The listing builds one solid part. Answer for the finished solid, in the listing's coordinates (mm). A direction names the side the tool comes from. Coordinates: 2 decimals unless noted, no trailing zeros. One line per item, written item: value. Start each with the question number.
```python
from build123d import *

# Parameters (mm, degrees)
SKETCH1_W           = 11.9
SKETCH1_H           = 5.95
BOSS_EXTRUDE1_DEPTH = 340
CUT_EXTRUDE1_DEPTH  = 341


with BuildPart() as part:
    # Sketch1 → Boss-Extrude1 (new body)
    with BuildSketch(Plane.XY):
        with BuildLine():
            Line((-4.350229073, 14.992640687), (-13.192640687, 14.992640687))
            ThreePointArc((-13.192640687, 14.992640687), (-14.465432893, 14.465432893), (-14.992640687, 13.192640687))
            Line((-14.992640687, 13.192640687), (-14.992640687, 4.350229073))
            Line((-14.992640687, 4.350229073), (-13.792640687, 4.350229073))
            ThreePointArc((-13.792640687, 4.350229073), (-13.085533906, 4.643122292), (-12.792640687, 5.350229073))
            Line((-12.792640687, 5.350229073), (-12.792640687, 8.460229073))
            Line((-12.792640687, 8.460229073), (-8.460229073, 8.460229073))
            Line((-8.460229073, 8.460229073), (-8.460229073, 12.792640687))
            Line((-8.460229073, 12.792640687), (-5.350229073, 12.792640687))
            ThreePointArc((-5.350229073, 12.792640687), (-4.643122292, 13.085533906), (-4.350229073, 13.792640687))
            Line((-4.350229073, 13.792640687), (-4.350229073, 14.992640687))
        make_face()
        with BuildLine():
            Line((-10.660229073, 13.792640687), (-12.792640687, 13.792640687))
            ThreePointArc((-12.792640687, 13.792640687), (-13.499747468, 13.499747468), (-13.792640687, 12.792640687))
            Line((-13.792640687, 12.792640687), (-13.792640687, 10.660229073))
            ThreePointArc((-13.792640687, 10.660229073), (-13.499747468, 9.953122292), (-12.792640687, 9.660229073))
            Line((-12.792640687, 9.660229073), (-10.660229073, 9.660229073))
            ThreePointArc((-10.660229073, 9.660229073), (-9.953122292, 9.953122292), (-9.660229073, 10.660229073))
            Line((-9.660229073, 10.660229073), (-9.660229073, 12.792640687))
            ThreePointArc((-9.660229073, 12.792640687), (-9.953122292, 13.499747468), (-10.660229073, 13.792640687))
        make_face(mode=Mode.SUBTRACT)
        Polygon((-5.95, 4.217588386), (-5.95, 5.95), (-4.217588386, 5.95), (-8.460229073, 10.192640687), (-8.460229073, 8.460229073), (-10.192640687, 8.460229073), align=None)
        with Locations((0, 2.975)):
            Rectangle(SKETCH1_W, SKETCH1_H)
        Polygon((8.460229073, 10.192640687), (4.217588386, 5.95), (5.95, 5.95), (5.95, 4.217588386), (10.192640687, 8.460229073), (8.460229073, 8.460229073), align=None)
        with BuildLine():
            Line((12.792640687, 8.460229073), (12.792640687, 5.350229073))
            ThreePointArc((12.792640687, 5.350229073), (13.085533906, 4.643122292), (13.792640687, 4.350229073))
            Line((13.792640687, 4.350229073), (14.992640687, 4.350229073))
            Line((14.992640687, 4.350229073), (14.992640687, 13.192640687))
            ThreePointArc((14.992640687, 13.192640687), (14.465432893, 14.465432893), (13.192640687, 14.992640687))
            Line((13.192640687, 14.992640687), (4.350229073, 14.992640687))
            Line((4.350229073, 14.992640687), (4.350229073, 13.792640687))
            ThreePointArc((4.350229073, 13.792640687), (4.643122292, 13.085533906), (5.350229073, 12.792640687))
            Line((5.350229073, 12.792640687), (8.460229073, 12.792640687))
            Line((8.460229073, 12.792640687), (8.460229073, 8.460229073))
            Line((8.460229073, 8.460229073), (12.792640687, 8.460229073))
        make_face()
        with BuildLine():
            ThreePointArc((9.660229073, 10.660229073), (9.953122292, 9.953122292), (10.660229073, 9.660229073))
            Line((10.660229073, 9.660229073), (12.792640687, 9.660229073))
            ThreePointArc((12.792640687, 9.660229073), (13.499747468, 9.953122292), (13.792640687, 10.660229073))
            Line((13.792640687, 10.660229073), (13.792640687, 12.792640687))
            ThreePointArc((13.792640687, 12.792640687), (13.499747468, 13.499747468), (12.792640687, 13.792640687))
            Line((12.792640687, 13.792640687), (10.660229073, 13.792640687))
            ThreePointArc((10.660229073, 13.792640687), (9.953122292, 13.499747468), (9.660229073, 12.792640687))
            Line((9.660229073, 12.792640687), (9.660229073, 10.660229073))
        make_face(mode=Mode.SUBTRACT)
    extrude(amount=-BOSS_EXTRUDE1_DEPTH)

    # Mirror1: part across plane


with BuildPart() as part_1:
    add(part.part)
    add(part.part.mirror(Plane(origin=(0, 0, -340), x_dir=(0, 0, 1), z_dir=(0, -1, 0))))

    # Sketch2 → Cut-Extrude1 (cut, through all)
    with BuildSketch(Plane.XY):
        with BuildLine():
            Line((-4.631549417, 3.075914498), (-3.16821753, 1.612582612))
            ThreePointArc((-3.16821753, 1.612582612), (-2.513764607, 2.513764607), (-1.612582612, 3.16821753))
            Line((-1.612582612, 3.16821753), (-3.075914498, 4.631549417))
            Line((-3.075914498, 4.631549417), (-4.631549417, 3.075914498))
        make_face()
        with BuildLine():
            Line((-3.16821753, 1.612582612), (-1.555634919, 0))
            Line((-1.555634919, 0), (0, 1.555634919))
            Line((0, 1.555634919), (-1.612582612, 3.16821753))
            ThreePointArc((-1.612582612, 3.16821753), (-2.513764607, 2.513764607), (-3.16821753, 1.612582612))
        make_face()
        with BuildLine():
            ThreePointArc((-3.16821753, 1.612582612), (-3.555, 0), (-3.16821753, -1.612582612))
            Line((-3.16821753, -1.612582612), (-1.555634919, 0))
            Line((-1.555634919, 0), (-3.16821753, 1.612582612))
        make_face()
        with BuildLine():
            Line((-4.631549417, -3.075914498), (-3.075914498, -4.631549417))
            Line((-3.075914498, -4.631549417), (-1.612582612, -3.16821753))
            ThreePointArc((-1.612582612, -3.16821753), (-2.513764607, -2.513764607), (-3.16821753, -1.612582612))
            Line((-3.16821753, -1.612582612), (-4.631549417, -3.075914498))
        make_face()
        with BuildLine():
            ThreePointArc((-3.16821753, -1.612582612), (-2.513764607, -2.513764607), (-1.612582612, -3.16821753))
            Line((-1.612582612, -3.16821753), (0, -1.555634919))
            Line((0, -1.555634919), (-1.555634919, 0))
            Line((-1.555634919, 0), (-3.16821753, -1.612582612))
        make_face()
        with BuildLine():
            Line((0, -1.555634919), (-1.612582612, -3.16821753))
            ThreePointArc((-1.612582612, -3.16821753), (0, -3.555), (1.612582612, -3.16821753))
            Line((1.612582612, -3.16821753), (0, -1.555634919))
        make_face()
        with BuildLine():
            Line((1.555634919, 0), (0, -1.555634919))
            Line((0, -1.555634919), (1.612582612, -3.16821753))
            ThreePointArc((1.612582612, -3.16821753), (2.513764607, -2.513764607), (3.16821753, -1.612582612))
            Line((3.16821753, -1.612582612), (1.555634919, 0))
        make_face()
        with BuildLine():
            Line((3.16821753, 1.612582612), (1.555634919, 0))
            Line((1.555634919, 0), (3.16821753, -1.612582612))
            ThreePointArc((3.16821753, -1.612582612), (3.456952294, -0.829159719), (3.555, 0))
            ThreePointArc((3.555, 0), (3.456952294, 0.829159719), (3.16821753, 1.612582612))
        make_face()
        Polygon((-1.555634919, 0), (0, -1.555634919), (1.555634919, 0), (0, 1.555634919), align=None)
        with BuildLine():
            Line((0, 1.555634919), (1.555634919, 0))
            Line((1.555634919, 0), (3.16821753, 1.612582612))
            ThreePointArc((3.16821753, 1.612582612), (2.513764607, 2.513764607), (1.612582612, 3.16821753))
            Line((1.612582612, 3.16821753), (0, 1.555634919))
        make_face()
        with BuildLine():
            Line((-1.612582612, 3.16821753), (0, 1.555634919))
            Line((0, 1.555634919), (1.612582612, 3.16821753))
            ThreePointArc((1.612582612, 3.16821753), (0, 3.555), (-1.612582612, 3.16821753))
        make_face()
        with BuildLine():
            ThreePointArc((1.612582612, 3.16821753), (2.513764607, 2.513764607), (3.16821753, 1.612582612))
            Line((3.16821753, 1.612582612), (4.631549417, 3.075914498))
            Line((4.631549417, 3.075914498), (3.075914498, 4.631549417))
            Line((3.075914498, 4.631549417), (1.612582612, 3.16821753))
        make_face()
        with BuildLine():
            ThreePointArc((3.16821753, -1.612582612), (2.513764607, -2.513764607), (1.612582612, -3.16821753))
            Line((1.612582612, -3.16821753), (3.075914498, -4.631549417))
            Line((3.075914498, -4.631549417), (4.631549417, -3.075914498))
            Line((4.631549417, -3.075914498), (3.16821753, -1.612582612))
        make_face()
    extrude(amount=-CUT_EXTRUDE1_DEPTH, mode=Mode.SUBTRACT)


solid = part_1.part
```
(1) For a pull along Y with two mould halves and no side action, classify faces 1 (the face through (-5.95, 0, -168)), 2 (the face through (14.993, -9, -168)), 3 (the face through (0, 5.95, -168)) as pulls with the +Y half, pulls with the -Y half, needs draft (parallel to the pull), parting line crosses it, or undercut.
(2) Flat-ended cylindrical pins translate along their axes: pin 1 Ø0.6 at (x, z) = (14.5, -120.5) entering from +Y; pin 2 Ø4 at (x, z) = (-1, -210) entering from +Y; pin 3 Ø1 at (x, z) = (3.5, -290) entering from -Y. Find the tip coordinate at first contact, or state that the pin passes through.
(3) Consider probe 1 along X at (y, z) = (12, -102.5); probe 2 along Y at (x, z) = (2.75, -202.5). Determine where each line is inside the solid, lowest interval first.
(4) For faces 4 (the face through (5.95, 0, -168)), 5 (the face through (0, -5.95, -168)), 6 (the face through (-14.993, 9, -168)), determine the directions among +Z, -Z, +X, -X, +Y, -Y from which every point of the face is accessible in a straight line to the end or side of a thin tool.
(5) The part is cut by section A-A on z = -317.5. Count the separate pieces of the cut face and the enclosed holes in it, plus the area to 3 significant figures.
Completed:
1. face 1: undercut
1. face 2: needs draft
1. face 3: pulls with the +Y half
2. pin 1: stops at y = 14.68
2. pin 2: stops at y = 5.95
2. pin 3: stops at y = -5.95
3. probe 1: x = -14.99 to -13.79, -9.66 to -8.46, 8.46 to 9.66, 13.79 to 14.99
3. probe 2: y = -5.95 to -4.31, 4.31 to 5.95
4. face 4: +Z, -Z, +X
4. face 5: +Z, -Z, -Y
4. face 6: +Z, -Z, -X, +Y, -Y
5. separate pieces: 1
5. enclosed holes: 5
5. area: 305 mm2
